```python
from build123d import *

# Parameters (mm, degrees)
F0_W     = 76.00291
F0_H     = 68.219476
F1_DEPTH = 32
F3_DEPTH = 25


with BuildPart() as f1:
    # F0 (on Top) → F1 (new body, symmetric)
    with BuildSketch(Plane.XY):
        Rectangle(F0_W, F0_H)
    extrude(amount=F1_DEPTH, both=True)

    # F2 (on face) → F3 (cut)
    with BuildSketch(Plane.XY.offset(32)):
        Polygon((-38.001455, -34.109738), (38.001455, -34.109738), (38.001455, 16.062718), (-38.001455, -8.216379), align=None)
    extrude(amount=-F3_DEPTH, mode=Mode.SUBTRACT)


solid = f1.part
```
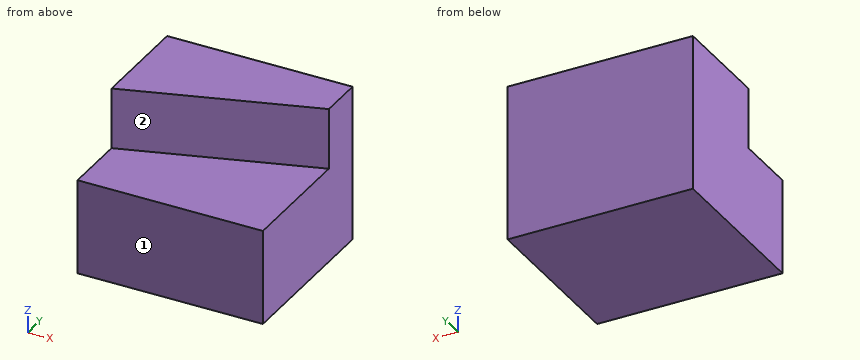
Can you work these out from the model? Positions are in its coordinate system, mm. Face numbers are marked on the shaded views. A direction names the side the tool comes from. Give positions to 0.01 mm unless a question says otherwise; leave off trailing zeros. Order: outer loops, then holes, each group sorted by start corner. A loop starts at its lowest first (then second) coordinate and runs counter-clockwise, first axis right, second up. Notation, with made-up numbers: (33.5, -17.5) - (59.5, -17.5) arc R34 ccw to (59.5, 18.5) - close; hole circle Ø7 at (-8, -35.5). An arc over 180 degrees is marked (long way). Use a Markdown table: item, result. Add a question column.
Q1. On a 3-axis mill with a long thin cutter (end or side, diameter ignored), from which of +Z, -Z, +X, -X, +Y, -Y can I reach the whole of each face in a straight line? I mean the marked faces 1 and 2. Say none if no direction works.
Q2. If we section it at A-A on y = -20.5: Write out the boundary of the cut face in (x, z), plus the area to 3 significant figures.
Q3. If we section it at B-B on z = 20: Write out the boundary of the cut face in (x, y), plus the area to 3 significant figures.
Q4. Please list where these lines run through material, in increasing order: line 1 along Z through (x, y) = (-19.5, -6); line 2 along Y through (x, z) = (10.5, 20.5); line 3 along Y through (x, z) = (-1.5, 24).
Q5. If we section it at D-D on y = -6: Write out the boundary of the cut face in (x, z), plus the area to 3 significant figures.
Q6. If we section it at C-C on x = 1: Write out the boundary of the cut face in (y, z).
Answers follow:
| question | item | result |
|---|---|---|
| 1 | face 1 | +Z, -Z, +X, -X, -Y |
| 1 | face 2 | +Z, +X, -Y |
| 2 | outline | (-38, -32) - (38, -32) - (38, 7) - (-38, 7) - close |
| 2 | area | 2,960 mm^2 |
| 3 | outline | (-38, -8.22) - (38, 16.06) - (38, 34.11) - (-38, 34.11) - close |
| 3 | area | 2,290 mm^2 |
| 4 | line 1 | z = -32 to 7 |
| 4 | line 2 | y = 7.28 to 34.11 |
| 4 | line 3 | y = 3.44 to 34.11 |
| 5 | outline | (-38, -32) - (38, -32) - (38, 7) - (-31.06, 7) - (-31.06, 32) - (-38, 32) - close |
| 5 | area | 3,140 mm^2 |
| 6 | outline | (-34.11, -32) - (34.11, -32) - (34.11, 32) - (4.24, 32) - (4.24, 7) - (-34.11, 7) - close |
